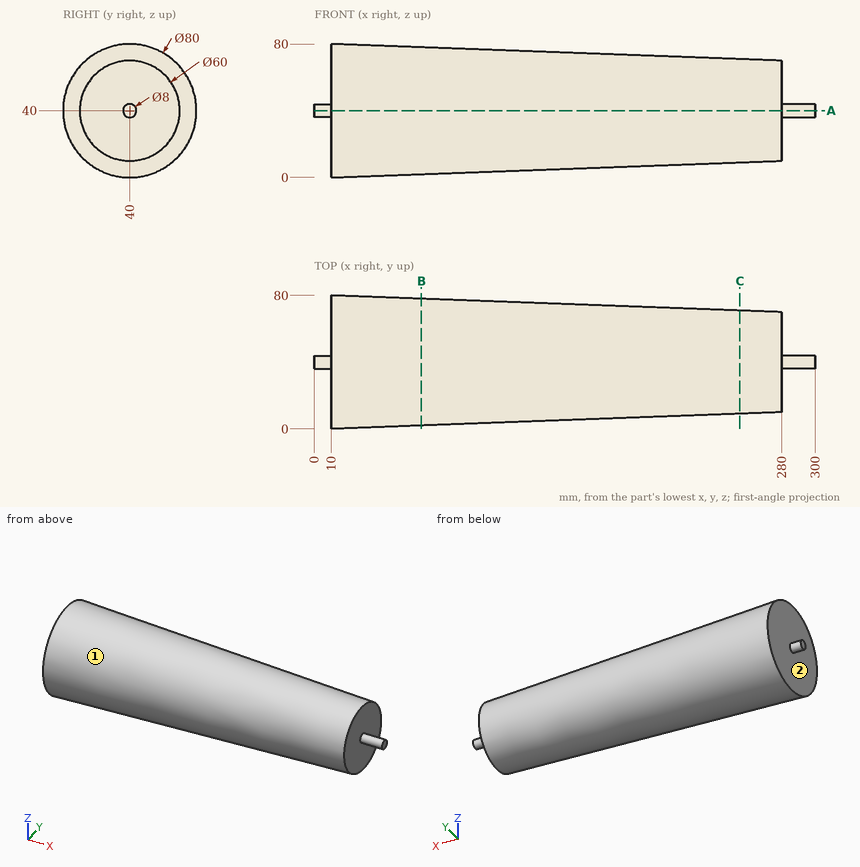
Print and shaded views of the part. All mm, measured from the part's lowest x, y and z. Round coordinates to 2 decimals unless told otherwise and drop trailing zeros. Order: outer loops, then holes, each group sorted by start corner. A loop starts at its lowest first (then second) coordinate and runs counter-clockwise, first axis right, second up.
Q1. Drop flat-ended pins along their axis: pin 1 (12 mm diameter, centred on y = 70.5, z = 32.5, fed in from +X); pin 2 (8 mm diameter, centred on x = 234, z = 44, fed in from +Y); pin 3 (1 mm diameter, centred on x = 176, y = 56.5, fed in from +Z). Give the stop position or say it passes through.
Q2. Wall check: L1, parallel to X at y = 39.5, z = 29.5; L2, parallel to Z at x = 29, y = 30; L3, parallel to Y at x = 117, z = 51.5. Give the ranges that are in metal, low to high.
Q3. Slice it at B-B (x = 64). Write the cut outline in (y, z).
Q4. Two-plate mould, pull along Y, no slides. Class the marked faces 1 and 2: pulls with the +Y half, pulls with the -Y half, needs draft (parallel to the pull), parting line crosses it, or undercut.
Q5. Slice it at C-C (x = 255). Write the cut outline in (y, z).
Q6. Slice it at A-A (z = 40). Write the cut outline in (x, y).
Results below:
1. pin 1: stops at x = 280
1. pin 2: stops at y = 71.79
1. pin 3: stops at z = 69.83
2. L1: x = 10 to 280
2. L2: z = 2 to 78
2. L3: y = 5.85 to 74.15
3. outline: circle Ø76 at (40, 40)
4. face 1: parting line crosses it
4. face 2: needs draft
5. outline: circle Ø61.85 at (40, 40)
6. outline: (0, 36) - (10, 36) - (10, 0) - (280, 10) - (280, 36) - (300, 36) - (300, 44) - (280, 44) - (280, 70) - (10, 80) - (10, 44) - (0, 44) - close
